Input: part model. Units: mm. Frame: model coordinates. A direction names the side the tool comes from. Give positions to 0.01 mm unless a question says otherwise; leave off trailing zeros. Loops run counter-clockwise (first coordinate to the right, second up) from the corner with the lowest first, then second, coordinate; pieces in that order, holes last. Notation, with made-up numbers: (48.25, -11.5) - (80.25, -11.5) arc R22 ccw to (80.25, 8.5) - close; hole circle Ø10 at (51, 80). An arc over 180 degrees is marked (long way). Answer as a JSON object with one key per item and string values.
from build123d import *

# Parameters (mm, degrees)
FILLET_R = 2.54


with BuildPart() as part:
    # Sketch → Revolution (revolve)
    with BuildSketch(Plane.XZ):
        Polygon((6.096, 0), (6.096, -6.477), (7.6835, -6.477), (7.6835, 0), (8.89, 7.6962), (7.3025, 7.6962), (1.5875, 1.5875), (1.5875, 0), align=None)
    revolve(axis=Axis((0, 0, 0), (0, 0, 1)))

    # Fillet
    fillet_edges = [part.edges().sort_by_distance(p)[0] for p in [
        (-1.5875, 0, 1.5875),
    ]]
    fillet(fillet_edges, radius=FILLET_R)


solid = part.part
Item 1: Cut plane A-A (z = -3). Return loops of the section in (x, y), then the cut area to 3 significant figures.
Geometry check:
{"outline": "circle Ø15.37 at (0, 0); hole circle Ø12.19 at (0, 0)", "area": "68.7 mm2"}
Item 2: Access query for faces 1 (the face through (-1.3, -1.3, 0)), 2 (the face through (-0.34, -1.55, 0.29)). Directions: +Z, -Z, +X, -X, +Y, -Y. A direction counts if a zero-diameter tool reaches every point of the face in a straight line with its end or side. Return the directions, or none.
Geometry check:
{"face 1": "-Z", "face 2": "+Z, -Z"}
Item 3: Cut plane B-B (z = 3.25). Return loops of the section in (x, y), then the cut area to 3 significant figures.
Geometry check:
{"outline": "circle Ø16.39 at (0, 0); hole circle Ø6.29 at (0, 0)", "area": "180 mm2"}
Item 4: Mould query, pull axis Y, two halves, no side actions, for faces 3 (the face through (-0.546, -2.457, 2.581)), 4 (the face through (5, 4, -6.477)), 5 (the face through (7.33, 2.31, -3.19)). Classes: released by +Y, released by -Y, zero draft, split by the parting line, or undercut.
Geometry check:
{"face 3": "undercut", "face 4": "zero draft", "face 5": "split by the parting line"}
Item 5: Material intervals for line 1 (Y direction, x = 0, z = -1.5); line 2 (X direction, y = 1, z = 5); line 3 (X direction, y = 1.75, z = -5), sorted ascending. Write a range as [from, to].
Geometry check:
{"line 1": "y = [-7.68, -6.1], [6.1, 7.68]", "line 2": "x = [-8.41, -4.67], [4.67, 8.41]", "line 3": "x = [-7.48, -5.84], [5.84, 7.48]"}
Item 6: Contact query for flat-ended pins moving along their axis: P1, Ø2, axis at x = -5, z = 1.5, coming from the -Y side; P2, Ø3, axis at x = -5, z = -4, coming from the +Y side; P3, Ø8, axis at x = -1, z = -1.5, coming from the +Y side. Output: stop coordinate, or through.
Geometry check:
{"P1": "stops at y = -6.86", "P2": "stops at y = 6.84", "P3": "stops at y = 8.06"}
